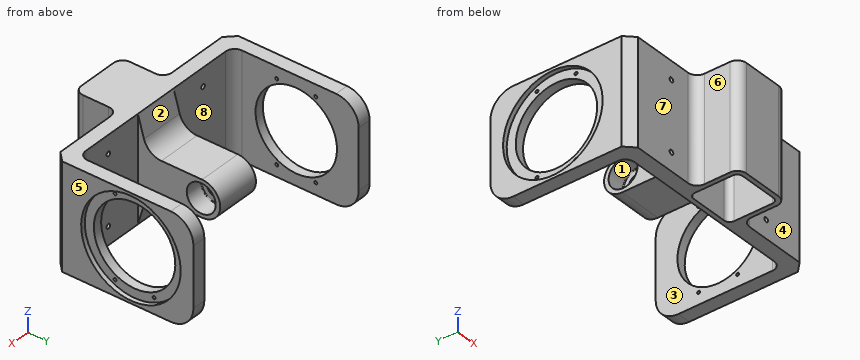
from build123d import *

# Parameters (mm, degrees)
BOSS_EXTRUDE1_DEPTH       = 116
SKETCH5_R                 = 16
CUT_EXTRUDE1_DEPTH        = 20
CUT_EXTRUDE2_REACH        = 6.51
SKETCH6_R                 = 10
CUT_EXTRUDE4_REACH        = 17
SKETCH8_R                 = 45
CUT_EXTRUDE5_DEPTH        = 106
FILLET3_R                 = 25
M6X1_0_TAPPED_HOLE1_D     = 5
M6X1_0_TAPPED_HOLE1_DEPTH = 16
SKETCH21_R                = 55
CUT_EXTRUDE7_DEPTH        = 5
M4X0_7_TAPPED_HOLE1_D     = 3.3
FILLET4_R                 = 0.8
CHAMFER1_SIZE             = 10
SKETCH25_W                = 64.356
SKETCH25_H                = 48.356
BOSS_EXTRUDE2_DEPTH       = 116
CUT_EXTRUDE8_DEPTH        = 106
FILLET6_R                 = 10
FILLET7_R                 = 10
FILLET8_R                 = 10


with BuildPart() as part:
    # Sketch1 → Boss-Extrude1 (new body)
    with BuildSketch(Plane.XY):
        Polygon((0, 0), (-106, 0), (-121, 0), (-121, 155), (-106, 155), (-106, 16), (-24.51, 16), (-24.51, 107), (0, 107), align=None)
    extrude(amount=-BOSS_EXTRUDE1_DEPTH)

    # Sketch5 → Cut-Extrude1 (cut)
    with BuildSketch(Plane.ZY.offset(24.51)):
        with Locations((-58, 86)):
            Circle(SKETCH5_R)
    extrude(amount=-CUT_EXTRUDE1_DEPTH, mode=Mode.SUBTRACT)

    # Sketch6 → Cut-Extrude2 (cut, up to next)
    with BuildSketch(Plane.ZY.offset(4.51), mode=Mode.PRIVATE) as cut_extrude2_sk1:
        with Locations((-58, 86)):
            Circle(SKETCH6_R)
    cut_extrude2_tool1 = extrude(cut_extrude2_sk1.sketch, amount=-CUT_EXTRUDE2_REACH, mode=Mode.PRIVATE) & part.part
    add(cut_extrude2_tool1.solids().sort_by_distance((-4.51, 86, -58))[0], mode=Mode.SUBTRACT)

    # Sketch8 → Cut-Extrude4 (cut, up to next)
    with BuildSketch(Plane(origin=(-106, 0, 0), x_dir=(0, 0, -1), z_dir=(1, 0, 0)), mode=Mode.PRIVATE) as cut_extrude4_sk1:
        with Locations((58, 86)):
            Circle(SKETCH8_R)
    cut_extrude4_tool1 = extrude(cut_extrude4_sk1.sketch, amount=-CUT_EXTRUDE4_REACH, mode=Mode.PRIVATE) & part.part
    add(cut_extrude4_tool1.solids().sort_by_distance((-106, 86, -58))[0], mode=Mode.SUBTRACT)

    # Sketch10 → Cut-Extrude5 (cut)
    with BuildSketch(Plane(origin=(0, 0, 0), x_dir=(0, 0, -1), z_dir=(1, 0, 0))):
        with BuildLine():
            Line((0, 107), (0, 16))
            Line((0, 16), (23.561161531, 22.820336233))
            ThreePointArc((23.561161531, 22.820336233), (33.987858372, 30.015449722), (38, 42.031621521))
            Line((38, 42.031621521), (38, 87))
            ThreePointArc((38, 87), (43.857864376, 101.142135624), (58, 107))
            Line((58, 107), (0, 107))
        make_face()
        with BuildLine():
            Line((116, 107), (58, 107))
            ThreePointArc((58, 107), (72.142135624, 101.142135624), (78, 87))
            Line((78, 87), (78, 42.031621521))
            ThreePointArc((78, 42.031621521), (82.012141628, 30.015449722), (92.438838469, 22.820336233))
            Line((92.438838469, 22.820336233), (116, 16))
            Line((116, 16), (116, 107))
        make_face()
    extrude(amount=-CUT_EXTRUDE5_DEPTH, mode=Mode.SUBTRACT)

    # Fillet3
    fillet3_edges = [part.edges().sort_by_distance(p)[0] for p in [
        (-113.5, 155, 0),
        (-113.5, 155, -116),
    ]]
    fillet(fillet3_edges, radius=FILLET3_R)

    # M6x1.0 Tapped Hole1
    with Locations(Plane(origin=(0, 0, 0), x_dir=(-1, 0, 0), z_dir=(0, -1, 0))):
        with Locations((65, 20), (65, 96)):
            Hole(M6X1_0_TAPPED_HOLE1_D / 2, depth=M6X1_0_TAPPED_HOLE1_DEPTH)

    # Sketch21 → Cut-Extrude7 (cut)
    with BuildSketch(Plane.ZY.offset(121)):
        with Locations((-58, 86)):
            Circle(SKETCH21_R)
    extrude(amount=-CUT_EXTRUDE7_DEPTH, mode=Mode.SUBTRACT)

    # M4x0.7 Tapped Hole1 (through all)
    with Locations(Plane.ZY.offset(116)):
        with Locations((-103.10855484, 107.568919311), (-12.89144516, 107.568919311), (-12.89144516, 64.431080689), (-103.10855484, 64.431080689)):
            Hole(M4X0_7_TAPPED_HOLE1_D / 2)

    # Mirror1: part across plane


with BuildPart() as part_1:
    add(part.part)
    add(part.part.mirror(Plane(origin=(0, 107, -116), x_dir=(0, 0, 1), z_dir=(1, 0, 0))))

    # Fillet4
    fillet4_edges = [part_1.edges().sort_by_distance(p)[0] for p in [
        (4.51, 86, -74),
        (-4.51, 86, -74),
    ]]
    fillet(fillet4_edges, radius=FILLET4_R)

    # Chamfer1
    chamfer1_edges = [part_1.edges().sort_by_distance(p)[0] for p in [
        (-121, 0, -58),
        (121, 0, -58),
    ]]
    chamfer(chamfer1_edges, length=CHAMFER1_SIZE)

    # Sketch25 → Boss-Extrude2 (add)
    with BuildSketch(Plane.XY):
        with Locations((0, -24.178)):
            Rectangle(SKETCH25_W, SKETCH25_H)
    extrude(amount=-BOSS_EXTRUDE2_DEPTH)

    # Sketch27 → Cut-Extrude8 (cut)
    with BuildSketch(Plane(origin=(0, 0, -116), x_dir=(-1, 0, 0), z_dir=(0, 0, -1))):
        with BuildLine():
            Line((-21.05025, -43.356), (21.05025, -43.356))
            ThreePointArc((21.05025, -43.356), (25.383223578, -41.561223578), (27.178, -37.22825))
            Line((27.178, -37.22825), (27.178, 4.87225))
            ThreePointArc((27.178, 4.87225), (25.383223578, 9.205223578), (21.05025, 11))
            Line((21.05025, 11), (-21.05025, 11))
            ThreePointArc((-21.05025, 11), (-25.383223578, 9.205223578), (-27.178, 4.87225))
            Line((-27.178, 4.87225), (-27.178, -37.22825))
            ThreePointArc((-27.178, -37.22825), (-25.383223578, -41.561223578), (-21.05025, -43.356))
        make_face()
    extrude(amount=-CUT_EXTRUDE8_DEPTH, mode=Mode.SUBTRACT)

    # Fillet6
    fillet6_edges = [part_1.edges().sort_by_distance(p)[0] for p in [
        (-32.178, 0, -58),
        (32.178, 0, -58),
    ]]
    fillet(fillet6_edges, radius=FILLET6_R)

    # Fillet7
    fillet7_edges = [part_1.edges().sort_by_distance(p)[0] for p in [
        (-32.178, -48.356, -58),
        (32.178, -48.356, -58),
    ]]
    fillet(fillet7_edges, radius=FILLET7_R)

    # Fillet8
    fillet8_edges = [part_1.edges().sort_by_distance(p)[0] for p in [
        (-106, 16, -58),
        (106, 16, -58),
    ]]
    fillet(fillet8_edges, radius=FILLET8_R)


solid = part_1.part
Design review of the part built by this model. Coordinates are the model's own, in mm. Face numbers are marked on the shaded views. A direction names the side the tool comes from. Round coordinates to 2 decimals unless told otherwise and drop trailing zeros. Loops run counter-clockwise (first coordinate to the right, second up) from the corner with the lowest first, then second, coordinate; pieces in that order, holes last. Notation, with made-up numbers: M -24.75,31.25 L -13.75,31.25 A24 cw -13.75,53.25 Z; hole C 2.5,38 d5. An arc over 180 degrees is marked long. Answer as a JSON object with one key per item and string values.
Item 1: We need section A-A on z = -58. State how many separate pieces and enclosed holes the cut face has, and give its area (3 significant figures).
Answer sheet:
{"separate pieces": "4", "enclosed holes": "1", "area": "8,280 mm^2"}
Item 2: The part is to be moulded in two halves that separate along X. For the marked faces 5, 6, 7 and 8, say which applies: pulls with the +X half, pulls with the -X half, needs draft (parallel to the pull), parting line crosses it, or undercut.
Answer sheet:
{"face 5": "pulls with the +X half", "face 6": "pulls with the -X half", "face 7": "needs draft", "face 8": "undercut"}
Item 3: Clearance check with flat-ended pins moving along their axes: P1, Ø5.5, axis at y = 107.57, z = -12.89, coming from the -X side; P2, Ø12, axis at x = -12, y = 38, coming from the +Z side; P3, Ø5, axis at y = -17.5, z = -85, coming from the -X side. State where each tip first meets the part, or that it passes through.
Answer sheet:
{"P1": "stops at x = -116", "P2": "stops at z = -35.3", "P3": "stops at x = -32.18"}
Item 4: Wall thickness on L1, parallel to X at y = 5, z = -96; L2, parallel to X at y = 128, z = -24; L3, parallel to X at y = -12, z = -68.5: over which ranges is each line inside the solid? List them lowest first. Write a range as from..to.
Answer sheet:
{"L1": "x = -116..-67.5, -62.5..-27.18, 27.18..62.5, 67.5..116", "L2": "x = -116..-106, 106..116", "L3": "x = -32.18..-27.18, 27.18..32.18"}
Item 5: We need section B-B on x = 89. Give the boundary of the cut face in (y, z).
Answer sheet:
{"outline": "M 0,-116 L 16,-116 L 16,0 L 0,0 Z"}
Item 6: Machinability: for the marked faces 1, 2, 3 and 4, which of the approach directions +Z, -Z, +X, -X, +Y, -Y give a long, thin tool a straight path to every point of the face, cutting with its end or side? Answer none if there is none.
Answer sheet:
{"face 1": "-X", "face 2": "+Z, +Y", "face 3": "+Z, -Z, +Y", "face 4": "+Z, -Z, +X, -Y"}
